Autodesk Inventor part; units mm, degrees
ref_plane "YZ Plane" through (0, 0, 0) normal (1, 0, 0) x (0, 1, 0)
ref_plane "XZ Plane" through (0, 0, 0) normal (0, 1, 0) x (-1, 0, 0)
ref_plane "XY Plane" through (0, 0, 0) normal (0, 0, 1) x (1, 0, 0)
sketch "Sketch1" plane through (0, 0, 0) normal (1, 0, 0) x (0, 1, 0)
  line L0 (3.175, 6.35) -> (-3.175, 6.35) construction
  line L1 (-3.175, 6.35) -> (-3.175, -6.35) construction
  line L2 (-3.175, -6.35) -> (3.175, -6.35) construction
  line L3 (3.175, -6.35) -> (3.175, 6.35) construction
  line L4 (3.175, 6.35) -> (-3.175, -6.35) construction
  line L5 (-3.175, 6.35) -> (3.175, -6.35) construction
  circle A0 centre (0, 0) radius 1.5
  circle A1 centre (3.175, 6.35) radius 1.5
  circle A2 centre (3.175, -6.35) radius 1.5
  circle A3 centre (-3.175, 6.35) radius 1.5
  circle A4 centre (-3.175, -6.35) radius 1.5
  line L6 (6.35, 22.225) -> (-6.35, 22.225)
  line L7 (-6.35, 22.225) -> (-6.35, -22.225)
  line L8 (-6.35, -22.225) -> (6.35, -22.225)
  line L9 (6.35, -22.225) -> (6.35, 22.225)
  line L10 (6.35, 22.225) -> (-6.35, -22.225) construction
  line L11 (-6.35, 22.225) -> (6.35, -22.225) construction
  line L12 (-6.35, 0) -> (6.35, 0) construction
  line L13 (-6.35, -3.175) -> (6.35, -3.175)
  line L14 (6.35, 3.175) -> (-6.35, 3.175)
  arc A5 (-6.35, 3.175) -> (-6.35, -3.175) centre (-6.35, 0) ccw
  arc A6 (6.35, -3.175) -> (6.35, 3.175) centre (6.35, 0) ccw
  circle A7 centre (3.175, 19.05) radius 1.5
  arc A8 (3.175, 22.225) -> (0.3352, 20.4699) centre (3.175, 19.05) ccw
  arc A9 (-6.0148, 7.7699) -> (-6.35, 6.35) centre (-3.175, 6.35) ccw
  line L15 (0.3352, 20.4699) -> (-6.0148, 7.7699)
  circle A10 centre (3.175, -19.05) radius 1.5
  arc A11 (0.3352, -20.4699) -> (3.175, -22.225) centre (3.175, -19.05) ccw
  arc A12 (-6.35, -6.35) -> (-6.0148, -7.7699) centre (-3.175, -6.35) ccw
  line L16 (0.3352, -20.4699) -> (-6.0148, -7.7699)
  point P0 (3.175, -22.225)
  point P1 (-6.35, -6.35)
  dimension "d0" = 6.35
  dimension "d1" = 12.7
  dimension "d2" = 3
  dimension "d3" = 3
  dimension "d6" = 12.7
  dimension "d9" = 6.35
  dimension "d12" = 12.7
  dimension "d13" = 44.45
  dimension "d14" = 6.35
  dimension "d20" = 3
  dimension "d21" = 12.7
extrude "Extrusion2" add sketch "Sketch1" against normal blind 3.175 contours L9 L14 L7 A9 L15 A8 L6 | L9 L13 L7 L14 | L9 L8 A11 L16 A12 L7 L13
equation "\"d6\" = d1"
equation "\"d9\" = d0"
properties part number "Pin Cap" material "Aluminum 6061"
Read the model definition and answer for the solid it produces. Units are mm, in the model's axes. Coordinates: 2 decimals unless noted, no trailing zeros. Write each loop counter-clockwise with the first axis right and the second up, starting at its lowest first coordinate (ties: lowest second). Pieces come first, ordered by that corner, then holes. Notation, with made-up numbers: (-22.75, 51) -> (29.25, 51) arc R24 ccw to (29.25, 69) -> close; hole circle Ø4 at (41, 38.25). An arc over 180 degrees is marked (long way). Answer as a JSON object with one key per item and string values.
Q1. Consider line 1 (Z direction, x = -2.85, y = 3); line 2 (Z direction, x = -0.95, y = 4) (3 decimals); line 3 (Y direction, x = -1.25, z = 18). Determine where each line is inside the solid, lowest interval first. Write a range as [from, to].
The answers:
{"line 1": "z = [-22.22, -20.54], [-17.56, -7.84], [-4.86, 4.86], [7.84, 17.56], [20.54, 22.22]", "line 2": "z = [-22.225, -20.303], [-17.797, -7.603], [-5.097, 5.097], [7.603, 17.797], [20.303, 22.225]", "line 3": "y = [-0.9, 2.1], [4.25, 6.35]"}
Q2. The part is cut by section C-C on z = 5.5. Give the vertices of the cut face in (x, y) (3 decimals).
The answers:
{"outline": "(-3.175, -6.35) -> (0, -6.35) -> (0, -4.411) -> (-3.175, -4.411) -> close; (-3.175, -1.939) -> (0, -1.939) -> (0, 1.939) -> (-3.175, 1.939) -> close; (-3.175, 4.411) -> (0, 4.411) -> (0, 6.35) -> (-3.175, 6.35) -> close"}
Q3. The part is cut by section D-D on y = 4.25. Give the vertices of the cut face in (x, z) (3 decimals), then the cut area to 3 significant figures.
The answers:
{"outline": "(-3.175, -22.225) -> (0, -22.225) -> (0, -20.096) -> (-3.175, -20.096) -> close; (-3.175, -18.004) -> (0, -18.004) -> (0, -7.396) -> (-3.175, -7.396) -> close; (-3.175, -5.304) -> (0, -5.304) -> (0, 5.304) -> (-3.175, 5.304) -> close; (-3.175, 7.396) -> (0, 7.396) -> (0, 18.004) -> (-3.175, 18.004) -> close; (-3.175, 20.096) -> (0, 20.096) -> (0, 22.225) -> (-3.175, 22.225) -> close", "area": "115 mm2"}
Q4. Determine the mould class of faces 1 (the cylindrical face through (-1.565, -4.674, 6.416)), 2 (the cylindrical face through (-1.565, 1.485, -21.738)), 3 (the flat face through (-2, 5, -22.225)) for opening direction Y: pulls with the +Y half, pulls with the -Y half, needs draft (parallel to the pull), parting line crosses it, or undercut.
The answers:
{"face 1": "undercut", "face 2": "pulls with the -Y half", "face 3": "needs draft"}
Q5. The part is cut by section A-A on x = -1.2. Give the vertices of the cut face in (y, z) (3 decimals), then the cut area to 3 significant figures.
The answers:
{"outline": "(-6.35, -6.35) arc R3.175 ccw to (-6.015, -7.77) -> (0.335, -20.47) arc R3.175 ccw to (3.175, -22.225) -> (6.35, -22.225) -> (6.35, 22.225) -> (3.175, 22.225) arc R3.175 ccw to (0.335, 20.47) -> (-6.015, 7.77) arc R3.175 ccw to (-6.35, 6.35) -> close; hole circle Ø3 at (-3.175, -6.35); hole circle Ø3 at (-3.175, 6.35); hole circle Ø3 at (0, 0); hole circle Ø3 at (3.175, -19.05); hole circle Ø3 at (3.175, -6.35); hole circle Ø3 at (3.175, 6.35); hole circle Ø3 at (3.175, 19.05)", "area": "399 mm2"}
Q6. The part is cut by section B-B on z = 0. Give the vertices of the cut face in (x, y) (3 decimals), then the cut area to 3 significant figures.
The answers:
{"outline": "(-3.175, -6.35) -> (0, -6.35) -> (0, -1.5) -> (-3.175, -1.5) -> close; (-3.175, 1.5) -> (0, 1.5) -> (0, 6.35) -> (-3.175, 6.35) -> close", "area": "30.8 mm2"}
